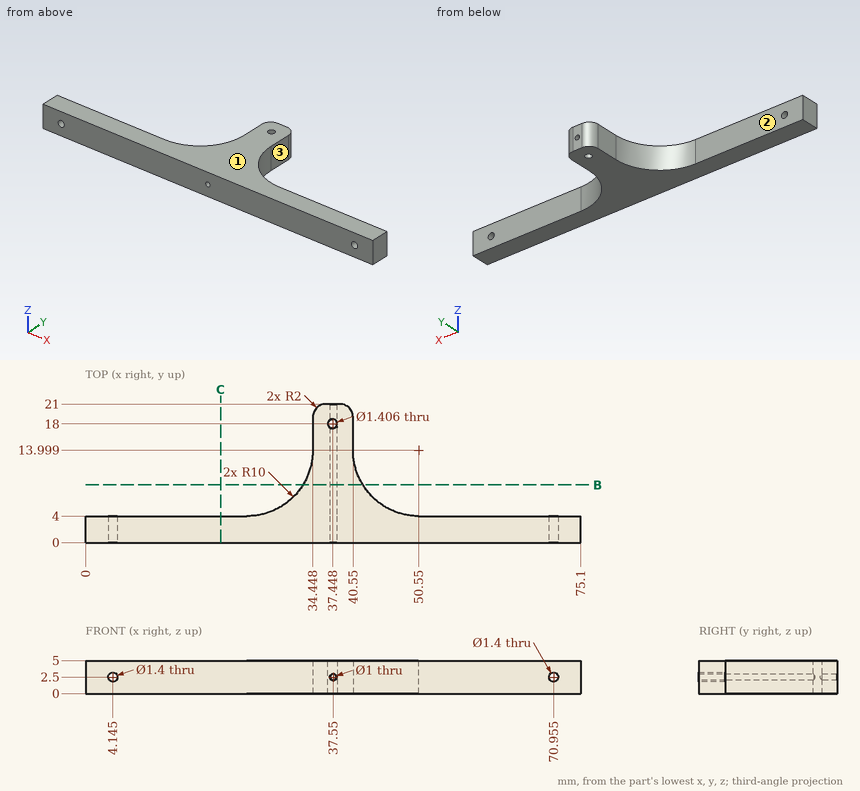
Part print with two shaded views. Sizes in mm from the minimum x, y, z corner. A direction names the side the tool comes from. Round coordinates to 2 decimals unless told otherwise and drop trailing zeros. Order: outer loops, then holes, each group sorted by start corner. A loop starts at its lowest first (then second) coordinate and runs counter-clockwise, first axis right, second up. Notation, with made-up numbers: (59, 30) -> (74, 30) arc R22 ccw to (74, 52) -> close; hole circle Ø2 at (4.5, 33). An arc over 180 degrees is marked (long way). Write each question's results on one line, items separated by ' | '.
1. Wall check: line 1 along X through (y, z) = (14.5, 2.5); line 2 along X through (y, z) = (19.2, 2.5); line 3 along Y through (x, z) = (23.5, 4.65). Give the ranges that are in metal, low to high. Write a range as [from, to].
Findings below:
line 1: x = [34.45, 37.05], [38.05, 40.55] | line 2: x = [34.46, 37.05], [38.05, 40.54] | line 3: y = [0, 4]
2. 3-axis set-ups, long thin cutter, end or side, ignore diameter. For the marked faces 1, 2 and 3: which of +Z, -Z, +X, -X, +Y, -Y reach the whole face in a straight line?
Findings below:
face 1: +Z, +X, -X, +Y, -Y | face 2: +Z, -Z, -X, +Y | face 3: +Z, -Z, +X, +Y
3. Flat gauge pins, fed straight in: P1, Ø1.8, axis at x = 70.955, z = 2.5, coming from the +Y side; P2, Ø2.5, axis at y = 15.5, z = 1.5, coming from the -X side. Where does each tip first touch, or does it go through?
Findings below:
P1: stops at y = 4 | P2: stops at x = 34.45
4. Cut at B-B (y = 8.75). Give the cut face in (x, z), plus the area to 3 significant figures.
Findings below:
outline: (32.96, 0) -> (42.04, 0) -> (42.04, 5) -> (32.96, 5) -> close; hole circle Ø1 at (37.55, 2.5) | area: 44.6 mm²
5. Cut at C-C (x = 20.5). Give the cut face in (y, z), plus the area to 3 significant figures.
Findings below:
outline: (0, 0) -> (4, 0) -> (4, 5) -> (0, 5) -> close | area: 20.0 mm²
